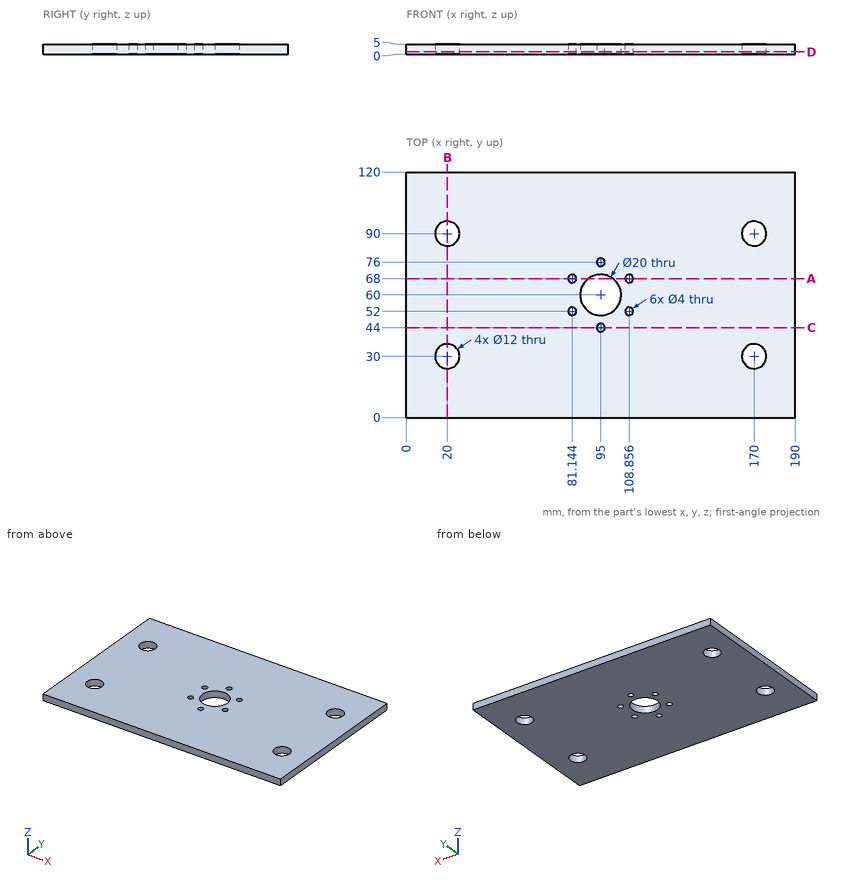
Check sheet for the drawn part. Datum: minimum x, y, z corner. Units: mm. Round coordinates to 2 decimals unless told otherwise and drop trailing zeros. Write each loop counter-clockwise with the first axis right and the second up, starting at its lowest first coordinate (ties: lowest second). Pieces come first, ordered by that corner, then holes. Notation, with made-up numbers: (48.25, 45) -> (76.25, 45) arc R20 cw to (76.25, 62) -> close; hole circle Ø2 at (88, -28). An arc over 180 degrees is marked (long way). Put each result on its own line as item: value.
(1) Sectioned sample at A-A (y = 68). Enter the section's corners in (x, z), plus the area to 3 significant figures.
Values found:
outline: (0, 0) -> (79.14, 0) -> (79.14, 5) -> (0, 5) -> close; (83.14, 0) -> (89, 0) -> (89, 5) -> (83.14, 5) -> close; (101, 0) -> (106.86, 0) -> (106.86, 5) -> (101, 5) -> close; (110.86, 0) -> (190, 0) -> (190, 5) -> (110.86, 5) -> close
area: 850 mm^2
(2) Sectioned sample at B-B (x = 20). Enter the section's corners in (y, z).
Values found:
outline: (0, 0) -> (24, 0) -> (24, 5) -> (0, 5) -> close; (36, 0) -> (84, 0) -> (84, 5) -> (36, 5) -> close; (96, 0) -> (120, 0) -> (120, 5) -> (96, 5) -> close
(3) Sectioned sample at D-D (z = 1.1). Count the separate pieces of the cut face and the enclosed holes in it, plus the area to 3 significant figures.
Values found:
separate pieces: 1
enclosed holes: 11
area: 22,000 mm^2
(4) Material ranges on line 1 (Y direction, x = 170, z = 2.15); line 2 (X direction, y = 27.5, z = 1.85) (1 decimal); line 3 (X direction, y = 68, z = 3.75) (1 decimal), recorded low to high.
Values found:
line 1: y = 0 to 24, 36 to 84, 96 to 120
line 2: x = 0 to 14.5, 25.5 to 164.5, 175.5 to 190
line 3: x = 0 to 79.1, 83.1 to 89, 101 to 106.9, 110.9 to 190
(5) Sectioned sample at C-C (y = 44). Enter the section's corners in (x, z).
Values found:
outline: (0, 0) -> (93, 0) -> (93, 5) -> (0, 5) -> close; (97, 0) -> (190, 0) -> (190, 5) -> (97, 5) -> close
